Can you work these out from the drawing? Everything is in mm from the part's minimum corner. A direction names the side the tool comes from. Round coordinates to 2 decimals unless told otherwise and drop trailing zeros. Loops run counter-clockwise (first coordinate to the right, second up) from the corner with the lowest first, then second, coordinate; pieces in that order, holes last. Notation, with made-up numbers: M 84.5,57.5 L 127.5,57.5 A10 ccw 127.5,67.5 Z; hole C 2,3 d3. An arc over 180 degrees is marked long. Answer in a Markdown table with one row per item.
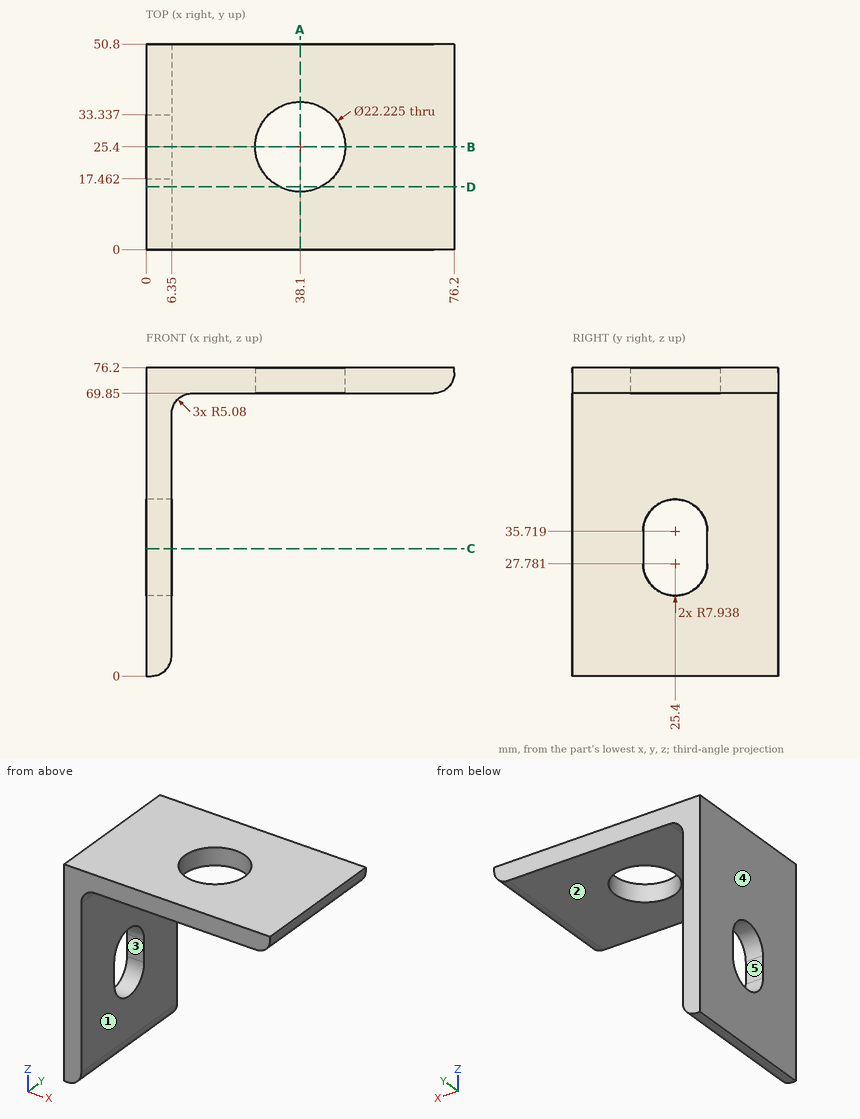
1) I want a section at D-D, the plane y = 15.5. Please give me the cut outline in (x, z).
Computed:
| item | result |
|---|---|
| outline | M 0,0 L 1.27,0 A5.08 ccw 6.35,5.08 L 6.35,64.77 A5.08 cw 11.43,69.85 L 33.05,69.85 L 33.05,76.2 L 0,76.2 Z; M 43.15,69.85 L 71.12,69.85 A5.08 ccw 76.2,74.93 L 76.2,76.2 L 43.15,76.2 Z |
2) Which directions (+Z, -Z, +X, -X, +Y, -Y) give clear straight access to the entire face, cutting with the end or side of a thin tool? Please do the marked faces 4 and 5.
Computed:
| item | result |
|---|---|
| face 4 | +Z, -Z, -X, +Y, -Y |
| face 5 | +X, -X |
3) Will these pins go through, and if not, where does the flat tip stop? P1, Ø12, axis at y = 30.5, z = 41, coming from the +X side; P2, Ø5, axis at x = 48.5, y = 15.5, coming from the -Z side; P3, Ø3, axis at x = 39.5, y = 17.5, coming from the +Z side; P4, Ø3, axis at y = 5.5, z = 19.5, coming from the +X side.
Computed:
| item | result |
|---|---|
| P1 | stops at x = 6.35 |
| P2 | stops at z = 69.85 |
| P3 | passes through |
| P4 | stops at x = 6.35 |
4) I want a section at B-B, the plane y = 25.4. Please give me the cut outline in (x, z).
Computed:
| item | result |
|---|---|
| outline | M 0,0 L 1.27,0 A5.08 ccw 6.35,5.08 L 6.35,19.84 L 0,19.84 Z; M 0,43.66 L 6.35,43.66 L 6.35,64.77 A5.08 cw 11.43,69.85 L 26.99,69.85 L 26.99,76.2 L 0,76.2 Z; M 49.21,69.85 L 71.12,69.85 A5.08 ccw 76.2,74.93 L 76.2,76.2 L 49.21,76.2 Z |
5) I want a section at A-A, the plane x = 38.1. Please give me the cut outline in (y, z).
Computed:
| item | result |
|---|---|
| outline | M 0,69.85 L 14.29,69.85 L 14.29,76.2 L 0,76.2 Z; M 36.51,69.85 L 50.8,69.85 L 50.8,76.2 L 36.51,76.2 Z |
6) I need wall thicknesses on line 1 (X direction, y = 25.4, z = 75); line 2 (Y direction, x = 38.1, z = 73.75); line 3 (Z direction, x = 57.5, y = 43). Which ranges of each line are inside material? Lowest first, please.
Computed:
| item | result |
|---|---|
| line 1 | x = 0 to 26.99, 49.21 to 76.2 |
| line 2 | y = 0 to 14.29, 36.51 to 50.8 |
| line 3 | z = 69.85 to 76.2 |
7) If we mould it in two halves opening along Z, with no side actions, what happens to the marked faces 1, 2 and 3? For each: released by +Z, released by -Z, zero draft, split by the parting line, or undercut.
Computed:
| item | result |
|---|---|
| face 1 | zero draft |
| face 2 | released by -Z |
| face 3 | undercut |
8) I want a section at C-C, the plane z = 31.5. Please give me the cut outline in (x, y), plus the area to 3 significant figures.
Computed:
| item | result |
|---|---|
| outline | M 0,0 L 6.35,0 L 6.35,17.46 L 0,17.46 Z; M 0,33.34 L 6.35,33.34 L 6.35,50.8 L 0,50.8 Z |
| area | 222 mm² |
